Geometry: final body of the model. Coordinates: model frame, mm. A direction names the side the tool comes from. Give positions to 0.01 mm unless a question says otherwise; leave off trailing zeros. Order: outer loops, then holes, each group sorted by start corner. A loop starts at its lowest first (then second) coordinate and runs counter-clockwise, first axis right, second up. Notation, with made-up numbers: (48, -26) -> (60, -26) arc R15 cw to (60, -9) -> close; hole circle Ø6 at (-20, 51). An arc over 180 degrees is marked (long way). One line per question, with ' | ' between items.
Autodesk Inventor part; units mm, degrees
ref_plane "YZ Plane" through (0, 0, 0) normal (1, 0, 0) x (0, 1, 0)
ref_plane "XZ Plane" through (0, 0, 0) normal (0, 1, 0) x (-1, 0, 0)
ref_plane "XY Plane" through (0, 0, 0) normal (0, 0, 1) x (1, 0, 0)
sketch "Эскиз1" plane through (0, 0, 0) normal (0, 0, 1) x (1, 0, 0)
  line L0 (0, 0) -> (-96, 0)
  line L1 (-96, 0) -> (-96, -96)
  line L2 (-96, -96) -> (0, -96)
  line L3 (0, -96) -> (0, 0)
  dimension "d0" = 96
  dimension "d1" = 96
extrude "Выдавливание1" add sketch "Эскиз1" along normal blind 11.5
fillet "Сопряжение1" radius 2 8 edges at (-48, 0, 11.5) (-96, -48, 11.5) (-96, 0, 5.75) (-96, -96, 5.75) (-48, -96, 11.5) (0, -48, 11.5) (0, -96, 5.75) (0, 0, 5.75)
sketch "Эскиз2" plane through (0, 0, 0) normal (0, 0, -1) x (-1, 0, 0)
  line L0 (2, -2) -> (94, -2)
  line L1 (94, -2) -> (94, -94)
  line L2 (94, -94) -> (2, -94)
  line L3 (2, -94) -> (2, -2)
  line L4 (18.852, -2) -> (35.4089, -2)
  line L5 (0, -94) -> (0, -2)
  line L6 (2, 0) -> (94, 0)
  point P0 (0, 0)
  dimension "d5" = 92
  dimension "d6" = 92
  dimension "d7" = 2
  dimension "d8" = 2
extrude "Выдавливание2" add sketch "Эскиз2" along normal blind 72
fillet "Сопряжение2" radius 2 8 edges at (-2, -2, -36) (-48, -2, -72) (-2, -48, -72) (-2, -94, -36) (-48, -94, -72) (-94, -94, -36) (-94, -48, -72) (-94, -2, -36)
sketch "Эскиз4" plane through (0, 0, 11.5) normal (0, 0, 1) x (1, 0, 0)
  line L0 (-88, -15) -> (-8, -15)
  line L1 (-8, -15) -> (-8, -60)
  line L2 (-8, -60) -> (-88, -60)
  line L3 (-88, -60) -> (-88, -15)
  line L4 (0, -94) -> (0, -2)
  line L5 (-2, 0) -> (-94, 0)
  point P0 (0, 0)
  dimension "d15" = 45
  dimension "d16" = 80
  dimension "d17" = 8
  dimension "d21" = 15
extrude "Выдавливание4" cut sketch "Эскиз4" against normal blind 1
fillet "Сопряжение3" radius 1 4 edges at (-8, -37.5, 11.5) (-48, -60, 11.5) (-48, -15, 11.5) (-88, -37.5, 11.5)
properties part number "EM20"
1) Set-up query: faces 5 (the flat face through (-94, -47, -35)), 6 (the flat face through (-49, -94, -35)), 7 (the flat face through (-47, -2, -35)). Return all of +Z, -Z, +X, -X, +Y, -Y with unobstructed straight access to the full face (end or side cutting, diameter ignored); none if empty.
Check result:
face 5: -Z, -X, +Y, -Y | face 6: -Z, +X, -X, -Y | face 7: -Z, +X, -X, +Y
2) Contact query for flat-ended pins moving along their axis: pin 1 Ø3 at (x, z) = (-43.5, -59.5) entering from -Y; pin 2 Ø10 at (y, z) = (-52.5, -2.5) entering from +X; pin 3 Ø6 at (x, y) = (-49, -56) entering from +Z; pin 4 Ø5 at (y, z) = (-63.5, -44) entering from -X. Output: stop coordinate, or through.
Check result:
pin 1: stops at y = -94 | pin 2: stops at x = 0 | pin 3: stops at z = 10.5 | pin 4: stops at x = -94
3) Section C-C on z = -43. Return loops of the section in (x, y), plus the area to 3 significant figures.
Check result:
outline: (-94, -92) arc R2 ccw to (-92, -94) -> (-4, -94) arc R2 ccw to (-2, -92) -> (-2, -4) arc R2 ccw to (-4, -2) -> (-92, -2) arc R2 ccw to (-94, -4) -> close | area: 8,460 mm^2
4) Pull-direction query (X, two-part tool) for faces 1 (the flat face through (-69.6, -1.6, 0)), 2 (the flat face through (-96, -47, 5)), 3 (the flat face through (-2, -49, -35)), 4 (the flat face through (-49, -37, 10.5)); classes: +X half, -X half, draft (parallel to the pull), parting line (faces both ways), or undercut.
Check result:
face 1: draft | face 2: -X half | face 3: +X half | face 4: undercut
5) Section D-D on y = -62.5. Return loops of the section in (x, z), plus the area to 3 significant figures.
Check result:
outline: (-96, 0) -> (-94, 0) -> (-94, -70) arc R2 ccw to (-92, -72) -> (-4, -72) arc R2 ccw to (-2, -70) -> (-2, 0) -> (0, 0) -> (0, 9.5) arc R2 ccw to (-2, 11.5) -> (-94, 11.5) arc R2 ccw to (-96, 9.5) -> close | area: 7,720 mm^2
6) Material intervals for probe 1 along Y at (x, z) = (-51, -33); probe 2 along Z at (x, y) = (-64.5, -16), sorted ascending. Write a range as from..to.
Check result:
probe 1: y = -94..-2 | probe 2: z = -72..10.5
